Autodesk Inventor part; units mm, degrees
ref_plane "YZ Plane" through (0, 0, 0) normal (1, 0, 0) x (0, 1, 0)
ref_plane "XZ Plane" through (0, 0, 0) normal (0, 1, 0) x (-1, 0, 0)
ref_plane "XY Plane" through (0, 0, 0) normal (0, 0, 1) x (1, 0, 0)
sketch "Sketch1" plane through (0, 0, 0) normal (0, 1, 0) x (-1, 0, 0)
  arc A0 (40.8631, 289.0847) -> (-143.2869, 104.9347) centre (40.8631, 104.9347) ccw
  line L0 (21.8131, 104.9347) -> (-143.2869, 104.9347)
  line L1 (40.8631, 289.0847) -> (40.8631, 123.9847)
  arc A1 (21.8131, 104.9347) -> (40.8631, 123.9847) centre (40.8631, 104.9347) ccw
  point P0 (0, 0)
  dimension "d0" = 368.3
  dimension "d2" = 0
  dimension "d3" = 38.1
extrude "Extrusion1" add sketch "Sketch1" along normal blind 3.175
sketch "Sketch2" plane through (0, 3.175, 0) normal (0, 1, 0) x (1, 0, 0)
  circle A0 centre (-30.9636, -95.0352) radius 1.25
  circle A1 centre (-30.9636, -114.8342) radius 1.25
  circle A2 centre (-50.7626, -114.8342) radius 1.25
  circle A3 centre (-50.7626, -95.0352) radius 1.25
  circle A4 centre (-50.7626, -114.8342) radius 0.996
  circle A5 centre (-30.9636, -114.8342) radius 0.996
  circle A6 centre (-30.9636, -95.0352) radius 0.996
  circle A7 centre (-50.7626, -95.0352) radius 0.996
  arc A8 (-21.8131, -104.9347) -> (-40.8631, -123.9847) centre (-40.8631, -104.9347) ccw
  circle A9 centre (-40.8631, -104.9347) radius 11.43
  point P0 (0, 0)
  dimension "d6" = 2.5
  dimension "d7" = 1.992
  dimension "d8" = 1.992
  dimension "d9" = 1.992
  dimension "d10" = 1.992
  dimension "d11" = 22.86
extrude "Extrusion2" cut sketch "Sketch2" against normal blind 3.175 contours A4 | A5 | A6 | A7 | A9
sketch "Sketch3" plane through (0, 3.175, 0) normal (0, 1, 0) x (1, 0, 0)
  arc A0 (-40.8631, -289.0847) -> (143.2869, -104.9347) centre (-40.8631, -104.9347) ccw
  circle A1 centre (-40.8631, -104.9347) radius 185.7375
  line L0 (143.2869, -104.9347) -> (144.8744, -104.9347)
  line L1 (-40.8631, -123.9847) -> (-40.8631, -289.0847)
  line L2 (-40.8631, -289.0847) -> (-40.8631, -290.6722)
  point P0 (0, 0)
  dimension "d14" = 184.15
  dimension "d15" = 371.475
extrude "Extrusion3" add sketch "Sketch3" along normal blind 25.4 and the other way blind 3.175 contours A0 L0 A1 L2 picked at (143.7515, -117.0198)
properties part number "ramp"
Source: CAD feature listing. Evaluate the final solid. Frame: model axes, mm. A direction names the side the tool comes from. Coordinates: 2 decimals unless noted, no trailing zeros. Loops run counter-clockwise (first coordinate to the right, second up) from the corner with the lowest first, then second, coordinate; pieces in that order, holes last. Notation, with made-up numbers: M -36,25 L -6,25 A23 ccw -6,55 Z; hole C 43,85 d4. An arc over 180 degrees is marked long. Use CSV: the item, a comma, the result in double quotes.
(1) Draft query along X for faces 6 (the face through (-54.77, 1.565, 91.916)), 7 (the face through (-49.934, 1.61, 111.89)), 8 (the face through (91.91, 14.09, 234.82)). Return one class per face: pulls with the +X half, pulls with the -X half, needs draft (parallel to the pull), parting line crosses it, or undercut.
Answers follow:
face 6,"parting line crosses it"
face 7,"undercut"
face 8,"pulls with the +X half"
(2) Reachability of faces 1 (the face through (44, 0, 190)), 2 (the face through (86, 28.575, 239)), 3 (the face through (90.774, 15.697, 233.709)), 4 (the face through (61, 2, 104.935)), 5 (the face through (-40.863, 2, 208)) from +Z, -Z, +X, -X, +Y, -Y: full face, straight path, thin tool, end or side. Return the list, or none.
Answers follow:
face 1,"+Z, -Z, +X, -X, -Y"
face 2,"+Z, -Z, +X, -X, +Y"
face 3,"-Z, -X, +Y"
face 4,"-Z, +X, +Y, -Y"
face 5,"+Z, -X, +Y, -Y"
(3) Cut plane A-A on x = 22. Return loops of the section in (y, z) (3 decimals), and give its area (3 significant figures).
Answers follow:
outline,"M 0,104.935 L 3.175,104.935 L 3.175,278.023 L 28.575,278.023 L 28.575,279.711 L 0,279.711 Z"
area,"598 mm²"
(4) Line query: line 1 (Z direction, x = -40, y = 13); line 2 (Y direction, x = 43, z = 263.5) (3 decimals); line 3 (Z direction, x = 50.5, y = 22). Output: solid intervals per line, ascending. Write a range as [from, to].
Answers follow:
line 1,"[289.08, 290.67]"
line 2,"[0, 3.175]"
line 3,"[264.82, 266.65]"
(5) Contact query for flat-ended pins moving along their axis: pin 1 (2.5 mm diameter, centred on x = -30.96, z = 95.04, fed in from -Y); pin 2 (6 mm diameter, centred on y = 16.5, z = 193, fed in from -X); pin 3 (12 mm diameter, centred on x = -11.5, y = 19, fed in from +Z); pin 4 (1 mm diameter, centred on x = 65.5, y = 19.5, fed in from -Z). Output: stop coordinate, or through.
Answers follow:
pin 1,"y = 0"
pin 2,"x = 119.19"
pin 3,"z = 289.2"
pin 4,"z = 254.91"
(6) Cut plane B-B on z = 254. Return loops of the section in (x, y) (3 decimals).
Answers follow:
outline,"M -40.863,0 L 69.943,0 L 69.943,28.575 L 67.261,28.575 L 67.261,3.175 L -40.863,3.175 Z"
